Here's how the part is built. I have some questions about the finished solid (model axes, mm). Round coordinates to 2 decimals unless told otherwise and drop trailing zeros. Write each loop counter-clockwise with the first axis right and the second up, starting at its lowest first coordinate (ties: lowest second). Pieces come first, ordered by that corner, then holes. Notation, with made-up numbers: (56, 76.5) -> (68, 76.5) arc R19 cw to (68, 107.5) -> close; hole circle Ø3 at (72, 36). An arc over 180 degrees is marked (long way). Answer as CSV lines item,"result".
Autodesk Inventor part; units mm, degrees
ref_plane "YZ Plane" through (0, 0, 0) normal (1, 0, 0) x (0, 1, 0)
ref_plane "XZ Plane" through (0, 0, 0) normal (0, 1, 0) x (-1, 0, 0)
ref_plane "XY Plane" through (0, 0, 0) normal (0, 0, 1) x (1, 0, 0)
sketch "Sketch1" plane through (0, 0, 0) normal (0, 1, 0) x (-1, 0, 0)
  line L0 (0, -135) -> (0, 190) construction
  line L1 (111, 0) -> (-155, 0) construction
  ellipse E0 centre (0, 0) end of major axis (0, 110) minor radius 80 construction
  arc A0 (79.5622, -11.4917) -> (91.5, 0) centre (80, 0) ccw
  arc A1 (0, -121.5) -> (11.4442, -108.8687) centre (0, -110) ccw
  arc A2 (53.6974, -81.5386) -> (66.0076, -62.1493) centre (60.3721, -72.1738) ccw
  arc A3 (79.5622, -11.4917) -> (66.0076, -62.1493) centre (79.2711, -38.556) ccw
  arc A4 (53.6974, -81.5386) -> (11.4442, -108.8687) centre (37.9882, -103.5791) ccw
  arc A5 (-91.5, 0) -> (-79.5622, -11.4917) centre (-80, 0) ccw
  arc A6 (-11.4442, -108.8687) -> (0, -121.5) centre (0, -110) ccw
  arc A7 (-66.0076, -62.1493) -> (-53.6974, -81.5386) centre (-60.3721, -72.1738) ccw
  arc A8 (-66.0076, -62.1493) -> (-79.5622, -11.4917) centre (-79.2711, -38.556) ccw
  arc A9 (-11.4442, -108.8687) -> (-53.6974, -81.5386) centre (-37.9882, -103.5791) ccw
  arc A10 (91.5, 0) -> (79.5622, 11.4917) centre (80, 0) ccw
  arc A11 (11.4442, 108.8687) -> (0, 121.5) centre (0, 110) ccw
  arc A12 (66.0076, 62.1493) -> (53.6974, 81.5386) centre (60.3721, 72.1738) ccw
  arc A13 (66.0076, 62.1493) -> (79.5622, 11.4917) centre (79.2711, 38.556) ccw
  arc A14 (11.4442, 108.8687) -> (53.6974, 81.5386) centre (37.9882, 103.5791) ccw
  arc A15 (0, 121.5) -> (-11.4442, 108.8687) centre (0, 110) ccw
  arc A16 (-53.6974, 81.5386) -> (-11.4442, 108.8687) centre (-37.9882, 103.5791) ccw
  arc A17 (-53.6974, 81.5386) -> (-66.0076, 62.1493) centre (-60.3721, 72.1738) ccw
  arc A18 (-79.5622, 11.4917) -> (-66.0076, 62.1493) centre (-79.2711, 38.556) ccw
  arc A19 (-79.5622, 11.4917) -> (-91.5, 0) centre (-80, 0) ccw
  line L2 (53.0109, -83.8154) -> (69.937, -57.0473) construction
  circle A20 centre (56.3638, -78.5129) radius 0.5
  line L3 (66.5644, -76.0894) -> (31.8982, -54.1692) construction
  circle A21 centre (64.3804, -65.8348) radius 0.5
  line L4 (80, -8.2711) -> (80, 9) construction
  circle A22 centre (80, -7.5) radius 0.5
  line L5 (9.0844, -110) -> (-9.2812, -110) construction
  circle A23 centre (7, -110) radius 0.5
  circle A24 centre (-56.3638, -78.5129) radius 0.5
  circle A25 centre (-64.3804, -65.8348) radius 0.5
  circle A26 centre (-80, -7.5) radius 0.5
  circle A27 centre (-7, -110) radius 0.5
  circle A28 centre (56.3638, 78.5129) radius 0.5
  circle A29 centre (64.3804, 65.8348) radius 0.5
  circle A30 centre (80, 7.5) radius 0.5
  circle A31 centre (7, 110) radius 0.5
  circle A32 centre (-7, 110) radius 0.5
  circle A33 centre (-56.3638, 78.5129) radius 0.5
  circle A34 centre (-64.3804, 65.8348) radius 0.5
  circle A35 centre (-80, 7.5) radius 0.5
  circle A36 centre (60.3721, -72.1738) radius 2
  circle A37 centre (0, -110) radius 2
  circle A38 centre (-60.3721, -72.1738) radius 2
  circle A39 centre (80, 0) radius 2
  circle A40 centre (-80, 0) radius 2
  circle A41 centre (60.3721, 72.1738) radius 2
  circle A42 centre (0, 110) radius 2
  circle A43 centre (-60.3721, 72.1738) radius 2
  line L6 (-12.5, 65) -> (-12.5, 74)
  circle A44 centre (50, 0) radius 1.75
  circle A45 centre (35.016, -56.1406) radius 1.75
  circle A46 centre (0, -80) radius 1.75
  circle A47 centre (-50, 0) radius 1.75
  circle A48 centre (-35.016, -56.1406) radius 1.75
  line L7 (66.5644, 76.0894) -> (31.8982, 54.1692) construction
  circle A49 centre (0, 110) radius 2
  circle A50 centre (35.016, 56.1406) radius 1.75
  circle A51 centre (0, 80) radius 1.75
  circle A52 centre (-35.016, 56.1406) radius 1.75
  dimension "d0" = 110
  dimension "d1" = 80
  dimension "d2" = 23
  dimension "d3" = 23
  dimension "d4" = 23
  dimension "d6" = 1
  dimension "d7" = 7.5
  dimension "d8" = 1
  dimension "d9" = 7.5
  dimension "d12" = 1
  dimension "d13" = 7
  dimension "d22" = 4
  dimension "d23" = 4
  dimension "d24" = 4
  dimension "d25" = 4
  dimension "d26" = 4
  dimension "d47" = 3.5
  dimension "d48" = 30
  dimension "d49" = 3.5
  dimension "d50" = 30
  dimension "d51" = 3.5
  dimension "d52" = 30
extrude "Extrusion7" add sketch "Sketch1" along normal blind 3
sketch "Sketch2" plane through (0, 0, 0) normal (0, -1, 0) x (1, 0, 0)
  line L0 (0, 96) -> (0, -64) construction
  line L1 (-60, 0) -> (61, 0) construction
  line L2 (-26.5, 15) -> (-25, 15)
  line L3 (-25, 15) -> (-25, 10)
  line L4 (-25, 10) -> (-26.5, 10)
  line L5 (-26.5, 10) -> (-26.5, 15)
  line L6 (-26.5, 35) -> (-25, 35)
  line L7 (-25, 35) -> (-25, 30)
  line L8 (-25, 30) -> (-26.5, 30)
  line L9 (-26.5, 30) -> (-26.5, 35)
  line L10 (26.5, 15) -> (25, 15)
  line L11 (25, 15) -> (25, 10)
  line L12 (25, 10) -> (26.5, 10)
  line L13 (26.5, 10) -> (26.5, 15)
  line L14 (26.5, 35) -> (25, 35)
  line L15 (25, 35) -> (25, 30)
  line L16 (25, 30) -> (26.5, 30)
  line L17 (26.5, 30) -> (26.5, 35)
  line L18 (-26.5, -15) -> (-25, -15)
  line L19 (-25, -15) -> (-25, -10)
  line L20 (-25, -10) -> (-26.5, -10)
  line L21 (-26.5, -10) -> (-26.5, -15)
  line L22 (-26.5, -35) -> (-25, -35)
  line L23 (-25, -35) -> (-25, -30)
  line L24 (-25, -30) -> (-26.5, -30)
  line L25 (-26.5, -30) -> (-26.5, -35)
  line L26 (26.5, -15) -> (25, -15)
  line L27 (25, -15) -> (25, -10)
  line L28 (25, -10) -> (26.5, -10)
  line L29 (26.5, -10) -> (26.5, -15)
  line L30 (26.5, -35) -> (25, -35)
  line L31 (25, -35) -> (25, -30)
  line L32 (25, -30) -> (26.5, -30)
  line L33 (26.5, -30) -> (26.5, -35)
  point P0 (0, 0)
  dimension "d57" = 1.5
  dimension "d58" = 5
  dimension "d59" = 25
  dimension "d60" = 10
  dimension "d61" = 1.5
  dimension "d62" = 5
  dimension "d63" = 30
extrude "Extrusion8" cut sketch "Sketch2" against normal blind 31.25
properties part number "BodyBottom"
1. Suppose I cut it at B-B on x = 30. Please give me the cut outline in (y, z).
Numbers:
outline,"(0, -77.72) -> (3, -77.72) -> (3, 77.72) -> (0, 77.72) -> close"
2. If I drill on line 1 (Z direction, x = -80, y = 2.8); line 2 (X direction, y = 1.15, z = 1); line 3 (X direction, y = 1.75, z = 33), over which ranges is the centre line in solid material (lowest first)?
Numbers:
line 1,"z = -11.5 to -8, -7 to -2, 2 to 7, 8 to 11.5"
line 2,"x = -91.46 to -81.73, -78.27 to -51.44, -48.56 to 48.56, 51.44 to 78.27, 81.73 to 91.46"
line 3,"x = -52.78 to -26.5, -25 to 25, 26.5 to 52.78"
3. If we mould it in two halves opening along Z, with no side actions, what happens to faces 1 (the face through (22.91, 1.48, 81.1)), 2 (the face through (87.882, 1.479, -8.374)), 3 (the face through (-69.938, 1.479, 78.557)), 4 (the face through (1, 0, 2))? For each: released by +Z, released by -Z, zero draft, split by the parting line, or undercut.
Numbers:
face 1,"undercut"
face 2,"released by -Z"
face 3,"undercut"
face 4,"zero draft"
4. For pin 1 Ø1.5 at (y, z) = (2, 32) entering from -X; pin 2 Ø0.8 at (x, y) = (26, 2) entering from -Z; pin 3 Ø1.5 at (y, z) = (0.5, 59.5) entering from -X, each with a flat end and sliding along its axis, tell me the tip position at first contact or that it passes through.
Numbers:
pin 1,"stops at x = -53.21"
pin 2,"stops at z = -79.51"
pin 3,"stops at x = -63.09"
5. Suppose I cut it at A-A on y = 1.05. Count the separate pieces of the cut face and the enclosed holes in it, and give its area (3 significant figures).
Numbers:
separate pieces,"1"
enclosed holes,"40"
area,"22,500 mm^2"
